Source: CAD feature listing. Evaluate the final solid. Frame: model axes, mm. A direction names the side the tool comes from. Give positions to 0.01 mm unless a question says otherwise; leave off trailing zeros. Order: outer loops, then holes, each group sorted by start corner. A loop starts at its lowest first (then second) coordinate and runs counter-clockwise, first axis right, second up. Notation, with made-up numbers: M 32,84.5 L 63,84.5 A23 cw 63,100.5 Z; hole C 12,34 d6. An arc over 180 degrees is marked long. Answer as a JSON object with one key per item and string values. Group by question number.
1. Section query A-A (z = 0). Output: boundary loops of the cut face in (x, y), plus the area to 3 significant figures.
2. Section query B-B (x = 0). Output: boundary loops of the cut face in (y, z).
3. Pin query (flat end, axial travel): P1, Ø1.6, axis at x = 0, y = -7, coming from the -Z side; P2, Ø1.5, axis at x = 2, z = 0.5, coming from the -Y side; P3, Ø1.6, axis at x = 0, y = -6, coming from the +Z side; P4, Ø1, axis at x = -1.5, z = 1.5, coming from the +Y side. Return the tip coordinate at first contact, or that it passes through.
4. Section query C-C (y = -1.5). Output: boundary loops of the cut face in (x, z).
5. Section query D-D (y = -5.75). Output: boundary loops of the cut face in (x, z).
6. Set-up query: faces 1 (the cylindrical face through (-1.45, -1.48, 0.06)), 2 (the flat face through (1, -6, 0)), 3 (the flat face through (-1, -6, 0)), 4 (the flat face through (0, -6, 2.5)), 5 (the flat face through (0, -6, -2.5)). Return all of +Z, -Z, +X, -X, +Y, -Y with unobstructed straight access to the full face (end or side cutting, diameter ignored); none if empty.
7. Material intervals for L1, parallel to Y at x = -2.55, z = -1.25; L2, parallel to X at y = -6.25, z = -0.05; L3, parallel to Y at x = 0.9, z = -1.8, sorted ascending. Write a range as [from, to].
from build123d import *

# Parameters (mm, degrees)
F0_R     = 1.45
F1_DEPTH = 3
F2_R     = 3
F3_DEPTH = 2.5
F4_R     = 0.9
F5_DEPTH = 1.98
F6_W     = 2
F6_H     = 5
F7_DEPTH = 2


with BuildPart() as f1:
    # F0 (on Front) → F1 (new body)
    with BuildSketch(Plane.XZ):
        Circle(F0_R)
    extrude(amount=F1_DEPTH)

    # F2 (on face) → F3 (join)
    with BuildSketch(Plane.XZ.offset(3)):
        Circle(F2_R)
    extrude(amount=F3_DEPTH)

    # F4 (on face) → F5 (join)
    with BuildSketch(Plane(origin=(0, 0, 0), x_dir=(-1, 0, 0), z_dir=(0, 1, 0))):
        Circle(F4_R)
    extrude(amount=F5_DEPTH)

    # F6 (on face) → F7 (join)
    with BuildSketch(Plane.XZ.offset(5.5)):
        Rectangle(F6_W, F6_H)
    extrude(amount=F7_DEPTH)


solid = f1.part
Answer sheet:
{
 "1": {"outline": "M -3,-5.5 L -1,-5.5 L -1,-7.5 L 1,-7.5 L 1,-5.5 L 3,-5.5 L 3,-3 L 1.45,-3 L 1.45,0 L 0.9,0 L 0.9,1.98 L -0.9,1.98 L -0.9,0 L -1.45,0 L -1.45,-3 L -3,-3 Z", "area": "31.3 mm^2"},
 "2": {"outline": "M -7.5,-2.5 L -5.5,-2.5 L -5.5,-3 L -3,-3 L -3,-1.45 L 0,-1.45 L 0,-0.9 L 1.98,-0.9 L 1.98,0.9 L 0,0.9 L 0,1.45 L -3,1.45 L -3,3 L -5.5,3 L -5.5,2.5 L -7.5,2.5 Z"},
 "3": {"P1": "z = -2.5", "P2": "y = -5.5", "P3": "z = 3", "P4": "y = -3"},
 "4": {"outline": "C 0,0 d2.9"},
 "5": {"outline": "M -1,-2.5 L 1,-2.5 L 1,2.5 L -1,2.5 Z"},
 "6": {"face 1": "+Y", "face 2": "+Z, -Z, +X, -Y", "face 3": "+Z, -Z, -X, -Y", "face 4": "+Z, +X, -X, -Y", "face 5": "-Z, +X, -X, -Y"},
 "7": {"L1": "[-5.5, -3]", "L2": "[-1, 1]", "L3": "[-7.5, -3]"}
}
